Design review of the part built by this model. Coordinates are the model's own, in mm. Give positions to 0.01 mm unless a question says otherwise; leave off trailing zeros. Loops run counter-clockwise (first coordinate to the right, second up) from the corner with the lowest first, then second, coordinate; pieces in that order, holes last.
Autodesk Inventor part; units mm, degrees
ref_plane "YZ Plane" through (0, 0, 0) normal (1, 0, 0) x (0, 1, 0)
ref_plane "XZ Plane" through (0, 0, 0) normal (0, 1, 0) x (-1, 0, 0)
ref_plane "XY Plane" through (0, 0, 0) normal (0, 0, 1) x (1, 0, 0)
sketch "Sketch1" plane through (0, 0, 0) normal (1, 0, 0) x (0, 1, 0)
  line L0 (-25, 25) -> (25, 25)
  line L1 (25, 25) -> (25, -25)
  line L2 (25, -25) -> (-25, -25)
  line L3 (-25, -25) -> (-25, 25)
  point P0 (0, 0)
  dimension "d0" = 50
  dimension "d1" = 50
  dimension "d2" = 25
  dimension "d3" = 25
extrude "Extrusion1" add sketch "Sketch1" along normal blind 6
sketch "Sketch2" plane through (6, 0, 0) normal (1, 0, 0) x (0, 0, -1)
  point P0 (0, 0)
  point P1 (0, 0)
hole "Hole1" at (6, 0, 0) direction (-1, 0, 0) diameter 4 end through all
fillet "Fillet1" radius 4 2 edges at (3, 25, 25) (3, 25, -25)
equation "\"d0\" = hoop_tabs_width"
equation "\"d1\" = hoop_tabs_width"
equation "\"d4\" = hoop_tabs_thickness"
equation "\"d6\" = hoop_tabs_hole"
equation "\"d13\" = hoop_tabs_hole"
equation "\"hoop_angle_z\" = 45deg"
equation "\"hoop_bearing_length\" = 5deg"
equation "\"hoop_cable_diam\" = 5"
equation "\"hoop_cable_pulley_diam\" = 22"
equation "\"rack_tooth_addendum\" = 5"
equation "\"rack_tooth_dedendum\" = 5"
equation "\"rack_tooth_thickness\" = 5"
equation "\"secure_arm_angle\" = 20deg"
equation "\"secure_arm_hold_length\" = 35"
equation "\"secure_arm_radii\" = 9"
equation "\"support_baseClamp_platformLengthBuffer\" = 35"
equation "\"support_baseClamp_platformThickness\" = 15"
equation "\"support_baseClamp_platformWidthBuffer\" = 0"
equation "\"support_baseClamp_sleeveHoleDiameter\" = 12"
equation "\"support_baseClamp_sleeveSweepTerminationAngle\" = 55deg"
equation "\"support_baseClamp_thickness\" = 8"
equation "\"support_frame_endHoleBuffer\" = 25"
equation "\"support_frame_squareBarFillet\" = 2"
equation "\"support_frame_squareBarThickness\" = 5"
equation "\"hoop_tabs_width\" = 50"
equation "\"hoop_tabs_thickness\" = 6"
equation "\"hoop_tabs_hole\" = 4"
properties part number "hoop_tab"
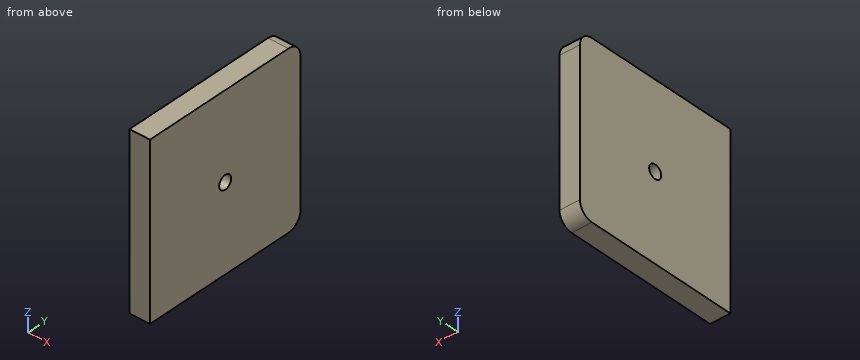
Q1. Take a section at A-A (y = 0). Give the boundary of the cut face in (x, z), plus the area to 3 significant figures.
Results:
outline: (0, -25) - (6, -25) - (6, -2) - (0, -2) - close; (0, 2) - (6, 2) - (6, 25) - (0, 25) - close
area: 276 mm2
Q2. Wall thickness on line 1 (Z direction, x = 4.45, y = 0); line 2 (Y direction, x = 0.3, z = 21.5): over which ranges is each line inside the solid? List them lowest first.
Results:
line 1: z = -25 to -2, 2 to 25
line 2: y = -25 to 24.97
